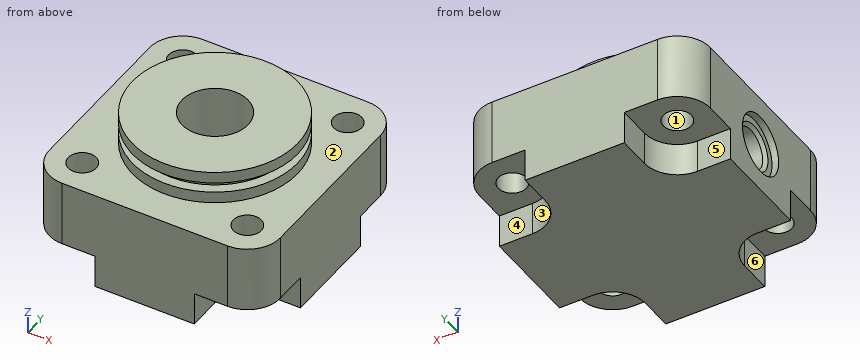
from build123d import *

# Parameters (mm, degrees)
SKETCH1_W               = 70
SKETCH1_H               = 70
BOSS_EXTRUDE1_DEPTH     = 30
SKETCH2_R               = 25
BOSS_EXTRUDE2_DEPTH     = 3.5
SKETCH3_R               = 22
BOSS_EXTRUDE3_DEPTH     = 3
SKETCH4_R               = 25
BOSS_EXTRUDE4_DEPTH     = 3.5
CUT_EXTRUDE1_REACH      = 65.64
SKETCH5_R               = 4.25
SKETCH5_3_W             = 20
SKETCH5_3_H             = 20
SKETCH5_3_R             = 4.25
CUT_EXTRUDE2_DEPTH      = 10
FILLET1_R               = 10
FILLET2_R               = 10
SKETCH7_R               = 10
CUT_EXTRUDE3_DEPTH      = 30
SKETCH8_R               = 9
CUT_EXTRUDE4_DEPTH      = 2
MIRROR6_COPY_1_REACH    = 65.64
MIRROR6_COPY_1_SKETCH_R = 4.25
MIRROR6_COPY_2_SKETCH_W = 20
MIRROR6_COPY_2_SKETCH_H = 20
MIRROR6_COPY_2_SKETCH_R = 4.25
MIRROR6_COPY_2_DEPTH    = 10
FILLET3_R               = 10
M14_TAPPED_HOLE1_D      = 12
M14_TAPPED_HOLE1_DEPTH  = 12
M14_TAPPED_HOLE1_TIP    = 3.605163714
CHAMFER1_SIZE           = 1
CUT_EXTRUDE5_REACH      = 88.308
CUT_EXTRUDE5_END_RADIUS = 10
SKETCH13_R              = 3


with BuildPart() as part:
    # Sketch1 → Boss-Extrude1 (new body)
    with BuildSketch(Plane.XY):
        Rectangle(SKETCH1_W, SKETCH1_H)
    extrude(amount=BOSS_EXTRUDE1_DEPTH)

    # Sketch2 → Boss-Extrude2 (add)
    with BuildSketch(Plane.XY.offset(30)):
        Circle(SKETCH2_R)
    extrude(amount=BOSS_EXTRUDE2_DEPTH)

    # Sketch3 → Boss-Extrude3 (add)
    with BuildSketch(Plane.XY.offset(33.5)):
        Circle(SKETCH3_R)
    extrude(amount=BOSS_EXTRUDE3_DEPTH)

    # Sketch4 → Boss-Extrude4 (add)
    with BuildSketch(Plane.XY.offset(36.5)):
        Circle(SKETCH4_R)
    extrude(amount=BOSS_EXTRUDE4_DEPTH)

    # Sketch5 → Cut-Extrude1 (cut, up to next)
    with BuildSketch(Plane(origin=(0, 0, 0), x_dir=(-1, 0, 0), z_dir=(0, 0, -1)), mode=Mode.PRIVATE) as cut_extrude1_sk1:
        with Locations((-25, 25)):
            Circle(SKETCH5_R)
    cut_extrude1_tool1 = extrude(cut_extrude1_sk1.sketch, amount=-CUT_EXTRUDE1_REACH, mode=Mode.PRIVATE) & part.part
    cut_extrude1 = cut_extrude1_tool1.solids().sort_by_distance((25, 25, 0))[0]
    add(cut_extrude1, mode=Mode.SUBTRACT)

    # Sketch5<3> → Cut-Extrude2 (cut)
    with BuildSketch(Plane(origin=(0, 0, 0), x_dir=(-1, 0, 0), z_dir=(0, 0, -1))):
        with Locations((-25, 25)):
            Rectangle(SKETCH5_3_W, SKETCH5_3_H)
        with Locations((-25, 25)):
            Circle(SKETCH5_3_R, mode=Mode.SUBTRACT)
    cut_extrude2 = extrude(amount=-CUT_EXTRUDE2_DEPTH, mode=Mode.SUBTRACT)

    # Fillet1
    fillet1_edges = [part.edges().sort_by_distance(p)[0] for p in [
        (15, 15, 5),
        (35, 35, 20),
    ]]
    fillet(fillet1_edges, radius=FILLET1_R)

    # Fillet2
    fillet2_edges = [part.edges().sort_by_distance(p)[0] for p in [
        (-35, 35, 15),
        (35, -35, 15),
        (-35, -35, 15),
    ]]
    fillet(fillet2_edges, radius=FILLET2_R)

    # Sketch7 → Cut-Extrude3 (cut)
    with BuildSketch(Plane.XY.offset(40)):
        Circle(SKETCH7_R)
    extrude(amount=-CUT_EXTRUDE3_DEPTH, mode=Mode.SUBTRACT)

    # Sketch8 → Cut-Extrude4 (cut)
    with BuildSketch(Plane.ZY.offset(35)):
        with Locations((15, 0)):
            Circle(SKETCH8_R)
    extrude(amount=-CUT_EXTRUDE4_DEPTH, mode=Mode.SUBTRACT)

    # Mirror5: Cut-Extrude1, Cut-Extrude2 across plane
    add(cut_extrude1.mirror(Plane.ZX), mode=Mode.SUBTRACT)
    add(cut_extrude2.mirror(Plane.ZX), mode=Mode.SUBTRACT)

    # Mirror6: Cut-Extrude1, Cut-Extrude2 across plane
    add(cut_extrude1.mirror(Plane(origin=(0, 0, 0), x_dir=(0, 0, 1), z_dir=(1, 0, 0))), mode=Mode.SUBTRACT)
    add(cut_extrude2.mirror(Plane(origin=(0, 0, 0), x_dir=(0, 0, 1), z_dir=(1, 0, 0))), mode=Mode.SUBTRACT)

    # Mirror6 copy 1 sketch → Mirror6 copy 1 (cut, up to next)
    with BuildSketch(Plane(origin=(0, 0, 0), x_dir=(1, 0, 0), z_dir=(0, 0, -1)), mode=Mode.PRIVATE) as mirror6_copy_1_sk1:
        with Locations((-25, 25)):
            Circle(MIRROR6_COPY_1_SKETCH_R)
    mirror6_copy_1_tool1 = extrude(mirror6_copy_1_sk1.sketch, amount=-MIRROR6_COPY_1_REACH, mode=Mode.PRIVATE) & part.part
    add(mirror6_copy_1_tool1.solids().sort_by_distance((-25, -25, 0))[0], mode=Mode.SUBTRACT)

    # Mirror6 copy 2 sketch → Mirror6 copy 2 (cut)
    with BuildSketch(Plane(origin=(0, 0, 0), x_dir=(1, 0, 0), z_dir=(0, 0, -1))):
        with Locations((-25, 25)):
            Rectangle(MIRROR6_COPY_2_SKETCH_W, MIRROR6_COPY_2_SKETCH_H)
        with Locations((-25, 25)):
            Circle(MIRROR6_COPY_2_SKETCH_R, mode=Mode.SUBTRACT)
    extrude(amount=-MIRROR6_COPY_2_DEPTH, mode=Mode.SUBTRACT)

    # Fillet3
    fillet3_edges = [part.edges().sort_by_distance(p)[0] for p in [
        (-15, 15, 5),
        (-15, -15, 5),
        (15, -15, 5),
    ]]
    fillet(fillet3_edges, radius=FILLET3_R)

    # M14 Tapped Hole1
    with Locations(Plane.ZY.offset(33)):
        with Locations((15, 0)):
            Hole(M14_TAPPED_HOLE1_D / 2, depth=M14_TAPPED_HOLE1_DEPTH)
            with Locations((0, 0, -(M14_TAPPED_HOLE1_DEPTH + M14_TAPPED_HOLE1_TIP / 2))):  # 118° drill point
                Cone(0, M14_TAPPED_HOLE1_D / 2, M14_TAPPED_HOLE1_TIP, mode=Mode.SUBTRACT)

    # Chamfer1
    chamfer1_edges = [part.edges().sort_by_distance(p)[0] for p in [
        (-33, 0, 21),
    ]]
    chamfer(chamfer1_edges, length=CHAMFER1_SIZE)

    # Cut-Extrude5: up to this cylinder (the profile starts outside it)
    cut_extrude5_end = Plane(origin=(0, 0, 15), z_dir=(0, 0, 1)) * Cylinder(CUT_EXTRUDE5_END_RADIUS, 197.616, mode=Mode.PRIVATE)
    # Sketch13 → Cut-Extrude5 (cut, up to the surface)
    with BuildSketch(Plane.ZY.offset(33), mode=Mode.PRIVATE) as cut_extrude5_sk1:
        with Locations((15, 0)):
            Circle(SKETCH13_R)
    cut_extrude5_tool1 = extrude(cut_extrude5_sk1.sketch, amount=-CUT_EXTRUDE5_REACH, mode=Mode.PRIVATE) - cut_extrude5_end
    add(cut_extrude5_tool1.solids().sort_by_distance((-33, 0, 15))[0], mode=Mode.SUBTRACT)


solid = part.part
Input: part model. Units: mm. Frame: model coordinates. Face numbers are marked on the shaded views. A direction names the side the tool comes from. Round coordinates to 2 decimals unless told otherwise and drop trailing zeros. Loops run counter-clockwise (first coordinate to the right, second up) from the corner with the lowest first, then second, coordinate; pieces in that order, holes last. Notation, with made-up numbers: (86.5, 4.25) -> (107.5, 4.25) arc R27 cw to (107.5, 36.25) -> close; hole circle Ø7 at (20.5, -6). An arc over 180 degrees is marked (long way). Answer as a JSON object with one key per item and string values. Group by question number.
1) Section query B-B on x = 27. Output: boundary loops of the cut face in (y, z), plus the area to 3 significant figures.
2) Pin query (flat end, axial travel): pin 1 (11 mm diameter, centred on y = 0, z = 15, fed in from -X); pin 2 (5.5 mm diameter, centred on y = 0, z = 15, fed in from -X); pin 3 (10 mm diameter, centred on x = 26, y = 27, fed in from -Z). Return the tip coordinate at first contact, or that it passes through.
3) Reachability of the marked faces 4, 5 and 6 from +Z, -Z, +X, -X, +Y, -Y: full face, straight path, thin tool, end or side. Return the list, or none.
4) Section query C-C on z = 23. Output: boundary loops of the cut face in (x, y), plus the area to 3 significant figures.
5) Section query A-A on z = 15. Output: boundary loops of the cut face in (x, y), plus the area to 3 significant figures.
6) Draft query along Y for the marked faces 1, 2 and 3. Return one class per face: +Y half, -Y half, draft (parallel to the pull), parting line (faces both ways), or undercut.
7) Section query D-D on y = 12. Output: boundary loops of the cut face in (x, z), plus the area to 3 significant figures.
8) Ray query, L1, parallel to Y at x = -25, z = 25; L2, parallel to Z at x = -27.75, y = 0; L3, parallel to Y at x = -26, z = 17.5. Return the intervals inside material, ascending.
Reply:
{
 "1": {"outline": "(-34.8, 10) -> (-28.75, 10) -> (-28.75, 30) -> (-34.8, 30) -> close; (-21.25, 10) -> (-15, 10) -> (-15, 0) -> (15, 0) -> (15, 10) -> (21.25, 10) -> (21.25, 30) -> (-21.25, 30) -> close; (28.75, 10) -> (34.8, 10) -> (34.8, 30) -> (28.75, 30) -> close", "area": "1,390 mm2"},
 "2": {"pin 1": "stops at x = -20.7", "pin 2": "stops at x = 9.61", "pin 3": "stops at z = 10"},
 "3": {"face 4": "-Z, +X, +Y", "face 5": "-Z, -X, +Y", "face 6": "-Z, -X, -Y"},
 "4": {"outline": "(-35, -25) arc R10 ccw to (-25, -35) -> (25, -35) arc R10 ccw to (35, -25) -> (35, 25) arc R10 ccw to (25, 35) -> (-25, 35) arc R10 ccw to (-35, 25) -> (-35, 4.12) -> (-33, 4.12) -> (-33, -4.12) -> (-35, -4.12) -> close; hole circle Ø8.5 at (-25, -25); hole circle Ø8.5 at (-25, 25); hole circle Ø20 at (0, 0); hole circle Ø8.5 at (25, -25); hole circle Ø8.5 at (25, 25)", "area": "4,260 mm2"},
 "5": {"outline": "(-35, -25) arc R10 ccw to (-25, -35) -> (25, -35) arc R10 ccw to (35, -25) -> (35, 25) arc R10 ccw to (25, 35) -> (-25, 35) arc R10 ccw to (-35, 25) -> (-35, 9) -> (-33, 9) -> (-33, 7) -> (-32, 6) -> (-21, 6) -> (-19.2, 3) -> (-9.54, 3) arc R10 cw (long way) to (-9.54, -3) -> (-19.2, -3) -> (-21, -6) -> (-32, -6) -> (-33, -7) -> (-33, -9) -> (-35, -9) -> close; hole circle Ø8.5 at (-25, -25); hole circle Ø8.5 at (-25, 25); hole circle Ø8.5 at (25, -25); hole circle Ø8.5 at (25, 25)", "area": "4,020 mm2"},
 "6": {"face 1": "undercut", "face 2": "draft", "face 3": "+Y half"},
 "7": {"outline": "(-35, 0) -> (35, 0) -> (35, 30) -> (21.93, 30) -> (21.93, 33.5) -> (18.44, 33.5) -> (18.44, 36.5) -> (21.93, 36.5) -> (21.93, 40) -> (-21.93, 40) -> (-21.93, 36.5) -> (-18.44, 36.5) -> (-18.44, 33.5) -> (-21.93, 33.5) -> (-21.93, 30) -> (-35, 30) -> close", "area": "2,520 mm2"},
 "8": {"L1": "y = -35 to -29.25, -20.75 to 20.75, 29.25 to 35", "L2": "z = 0 to 9, 21 to 30", "L3": "y = -34.95 to -29.13, -20.87 to -5.45, 5.45 to 20.87, 29.13 to 34.95"}
}
